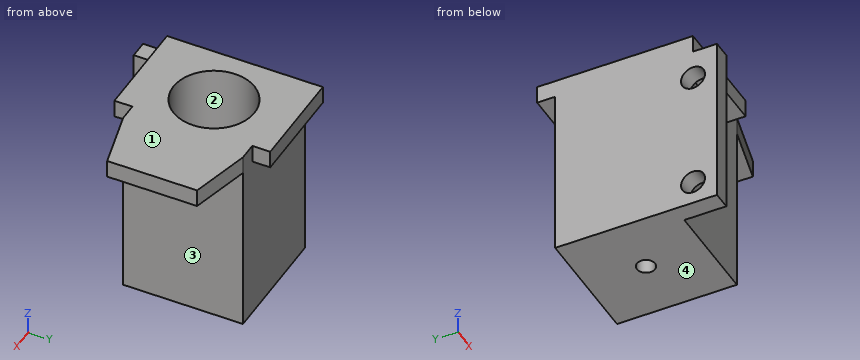
```python
from build123d import *

# Parameters (mm, degrees)
SKETCH_1_W          = 20
SKETCH_1_H          = 20
SKETCH_1_R          = 6.75
EXTRUDE_1_DEPTH     = 27
SKETCH_2_W          = 20
SKETCH_2_H          = 20
SKETCH_2_R          = 1.5
EXTRUDE_2_DEPTH     = 5
SKETCH_3_W          = 3
SKETCH_3_H          = 20
EXTRUDE_3_DEPTH     = 10
CUT_EXTRUDE_1_DEPTH = 10
SKETCH_5_W          = 17
SKETCH_5_H          = 3
EXTRUDE_4_DEPTH     = 3
SKETCH_7_W          = 29
SKETCH_7_H          = 7
EXTRUDE_5_DEPTH     = 3
SKETCH_8_R          = 2
CUT_EXTRUDE_2_DEPTH = 10


with BuildPart() as part:
    # 草图1 → 凸台-拉伸1 (new body)
    with BuildSketch(Plane.XY):
        Rectangle(SKETCH_1_W, SKETCH_1_H)
        Circle(SKETCH_1_R, mode=Mode.SUBTRACT)
    extrude(amount=EXTRUDE_1_DEPTH)

    # 草图2 → 凸台-拉伸2 (add)
    with BuildSketch(Plane(origin=(0, 0, 0), x_dir=(-1, 0, 0), z_dir=(0, 0, -1))):
        Rectangle(SKETCH_2_W, SKETCH_2_H)
        Circle(SKETCH_2_R, mode=Mode.SUBTRACT)
    extrude(amount=EXTRUDE_2_DEPTH)

    # 草图3 → 凸台-拉伸3 (add)
    with BuildSketch(Plane(origin=(10, 0, 0), x_dir=(0, 0, -1), z_dir=(1, 0, 0))):
        with Locations((-25.5, 0)):
            Rectangle(SKETCH_3_W, SKETCH_3_H)
    extrude(amount=EXTRUDE_3_DEPTH)

    # 草图4 → 切除-拉伸1 (cut)
    with BuildSketch(Plane(origin=(0, 0, 24), x_dir=(-1, 0, 0), z_dir=(0, 0, -1))):
        Polygon((-20, 7.5), (-10, 10), (-20, 10), align=None)
    cut_extrude_1 = extrude(amount=-CUT_EXTRUDE_1_DEPTH, mode=Mode.SUBTRACT)

    # 镜向1: 切除-拉伸1 across plane
    add(cut_extrude_1.mirror(Plane.ZX), mode=Mode.SUBTRACT)

    # 草图5 → 凸台-拉伸4 (add)
    with BuildSketch(Plane(origin=(0, 10, 0), x_dir=(1, 0, 0), z_dir=(0, 1, 0))):
        with Locations((-1.5, -25.5)):
            Rectangle(SKETCH_5_W, SKETCH_5_H)
    extrude_4 = extrude(amount=EXTRUDE_4_DEPTH)

    # 镜向2: 凸台-拉伸4 across plane
    add(extrude_4.mirror(Plane.ZX))

    # 草图7 → 凸台-拉伸5 (add)
    with BuildSketch(Plane.ZY.offset(10)):
        with Locations((9.5, -13.5)):
            Rectangle(SKETCH_7_W, SKETCH_7_H)
    extrude(amount=-EXTRUDE_5_DEPTH)

    # 草图8 → 切除-拉伸2 (cut)
    with BuildSketch(Plane.ZY.offset(10)):
        with Locations(Location((19, -13, 0), (0, 0, 270))):
            Circle(SKETCH_8_R)
        with Locations(Location((-1, -13, 0), (0, 0, 270))):
            Circle(SKETCH_8_R)
    extrude(amount=-CUT_EXTRUDE_2_DEPTH, mode=Mode.SUBTRACT)


solid = part.part
```
Design review of the part built by this model. Coordinates are the model's own, in mm. Face numbers are marked on the shaded views. A direction names the side the tool comes from. Give positions to 0.01 mm unless a question says otherwise; leave off trailing zeros. Write each loop counter-clockwise with the first axis right and the second up, starting at its lowest first coordinate (ties: lowest second). Pieces come first, ordered by that corner, then holes.
(1) Add section D-D (z = 9.5). Give the boundary of the cut face in (x, y).
Checked values:
outline: (-10, -17) - (-7, -17) - (-7, -10) - (10, -10) - (10, 10) - (-10, 10) - close; hole circle Ø13.5 at (0, 0)
(2) Mouldability with a two-part tool opening along Y and no side actions: class the marked faces 1 and 2 as +Y half, -Y half, draft (parallel to the pull), parting line (faces both ways), or undercut.
Checked values:
face 1: draft
face 2: undercut
(3) Add section A-A (z = 19). Give the boundary of the cut face in (x, y), and give its area (3 significant figures).
Checked values:
outline: (-10, -17) - (-7, -17) - (-7, -15) - (-10, -15) - close; (-10, -11) - (-7, -11) - (-7, -10) - (10, -10) - (10, 10) - (-10, 10) - close; hole circle Ø13.5 at (0, 0)
area: 266 mm2
(4) Clearance check with flat-ended pins moving along their axes: pin 1 Ø2 at (y, z) = (-12, 2.5) entering from +X; pin 2 Ø3.5 at (x, z) = (-1.5, 25) entering from -Y; pin 3 Ø3 at (y, z) = (-13, 19) entering from -X; pin 4 Ø1.5 at (y, z) = (-9.5, 10.5) entering from +X. State where each tip first meets the part, or that it passes through.
Checked values:
pin 1: stops at x = -7
pin 2: stops at y = -13
pin 3: passes through
pin 4: stops at x = 10
(5) Tool access review of the marked faces 3 and 4: name each direction out of +Z, -Z, +X, -X, +Y, -Y from which nothing blocks a thin tool from reaching the whole face with its end or side.
Checked values:
face 3: -Z, +X, +Y, -Y
face 4: -Z, +X, -X, +Y, -Y
(6) Add section B-B (y = 0). Give the boundary of the cut face in (x, z), and give its area (4 significant figures).
Checked values:
outline: (-10, -5) - (-1.5, -5) - (-1.5, 0) - (-6.75, 0) - (-6.75, 27) - (-10, 27) - close; (1.5, -5) - (10, -5) - (10, 24) - (20, 24) - (20, 27) - (6.75, 27) - (6.75, 0) - (1.5, 0) - close
area: 290.5 mm2
(7) Wall thickness on line 1 along X through (y, z) = (-14.5, 12); line 2 along Y through (x, z) = (0, -2.85); line 3 along Y through (x, z) = (-2.25, 17.5): over which ranges is each line inside the solid? List them lowest first.
Checked values:
line 1: x = -10 to -7
line 2: y = -10 to -1.5, 1.5 to 10
line 3: y = -10 to -6.36, 6.36 to 10
(8) Add section C-C (x = 0). Give the boundary of the cut face in (y, z), and give its area (4 significant figures).
Checked values:
outline: (-13, 24) - (-10, 24) - (-10, -5) - (-1.5, -5) - (-1.5, 0) - (-6.75, 0) - (-6.75, 27) - (-13, 27) - close; (1.5, -5) - (10, -5) - (10, 24) - (13, 24) - (13, 27) - (6.75, 27) - (6.75, 0) - (1.5, 0) - close
area: 278.5 mm2
